Geometry: see drawing. Coordinates: mm, zero at the bounding-box minimum. Round coordinates to 2 decimals unless told otherwise and drop trailing zeros. Loops run counter-clockwise (first coordinate to the right, second up) from the corner with the lowest first, then second, coordinate; pieces in that order, holes last.
(1) First-contact query: pin 1 Ø1.5 at (y, z) = (9.5, 2) entering from -X; pin 2 Ø2 at (y, z) = (6.5, 3.5) entering from -X; pin 3 Ø1.5 at (y, z) = (20.5, 7) entering from -X (1 decimal). Flat tips, straight axial feed; report the tip coordinate or a pass-through.
(2) Draft query along X for the marked faces 1, 2 and 3. Return one class per face: released by +X, released by -X, zero draft, split by the parting line, or undercut.
(3) Cut plane A-A, the plane y = 14. Output: boundary loops of the cut face in (x, z), and give its area (3 significant figures).
(4) Line query: line 1 (Y direction, x = 14, z = 2.75); line 2 (X direction, y = 13.75, z = 1.5) (1 decimal); line 3 (X direction, y = 8.5, z = 6.25) (1 decimal). Output: solid intervals per line, ascending.
(5) Cut plane C-C, the plane x = 14.25. Give the number of separate pieces and of enclosed holes in the cut face, and give its area (3 significant figures).
(6) Cut plane B-B, the plane z = 3. Output: boundary loops of the cut face in (x, y).
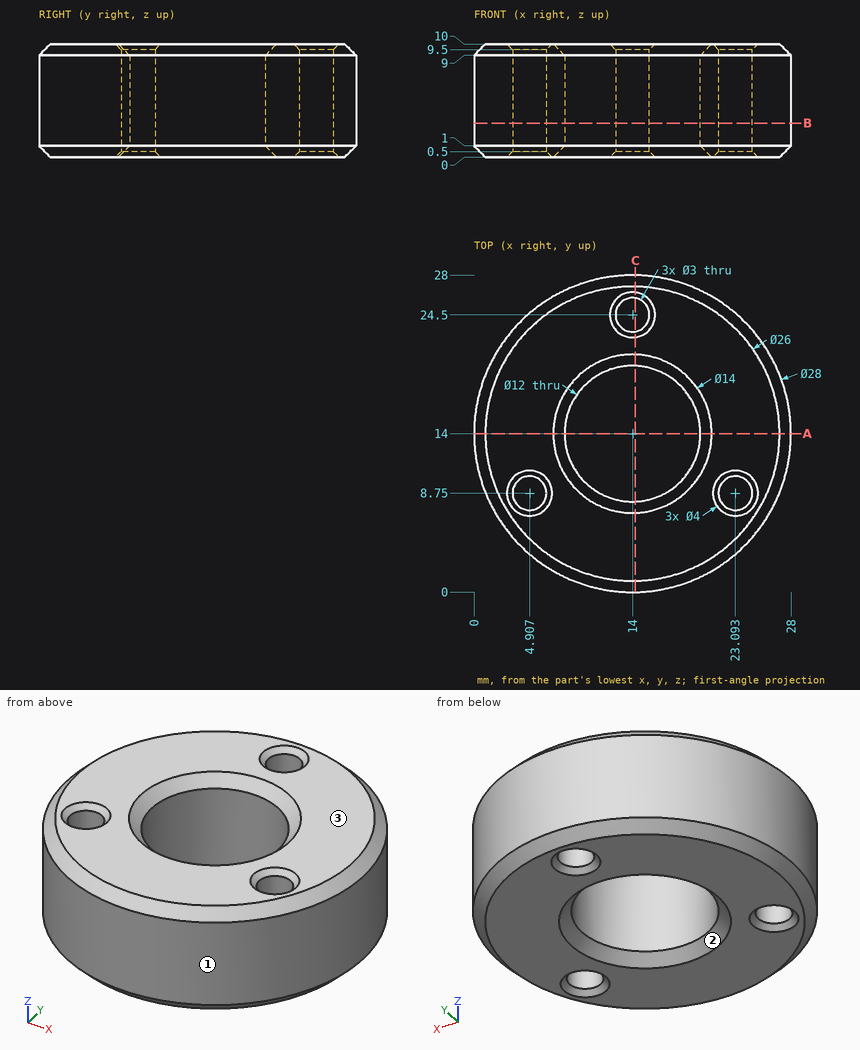
Reported:
1. pin 1: stops at x = 0.51
1. pin 2: stops at x = 1.6
1. pin 3: stops at x = 1.2
2. face 1: split by the parting line
2. face 2: undercut
2. face 3: zero draft
3. outline: (0, 1) - (1, 0) - (7, 0) - (8, 1) - (8, 9) - (7, 10) - (1, 10) - (0, 9) - close; (20, 1) - (21, 0) - (27, 0) - (28, 1) - (28, 9) - (27, 10) - (21, 10) - (20, 9) - close
3. area: 156 mm2
4. line 1: y = 0 to 8, 20 to 23, 26 to 28
4. line 2: x = 0 to 8, 20 to 28
4. line 3: x = 1.1 to 3.4, 6.4 to 11.6, 16.4 to 21.6, 24.6 to 26.9
5. separate pieces: 3
5. enclosed holes: 0
5. area: 126 mm2
6. outline: circle Ø28 at (14, 14); hole circle Ø3 at (4.91, 8.75); hole circle Ø12 at (14, 14); hole circle Ø3 at (14, 24.5); hole circle Ø3 at (23.09, 8.75)
